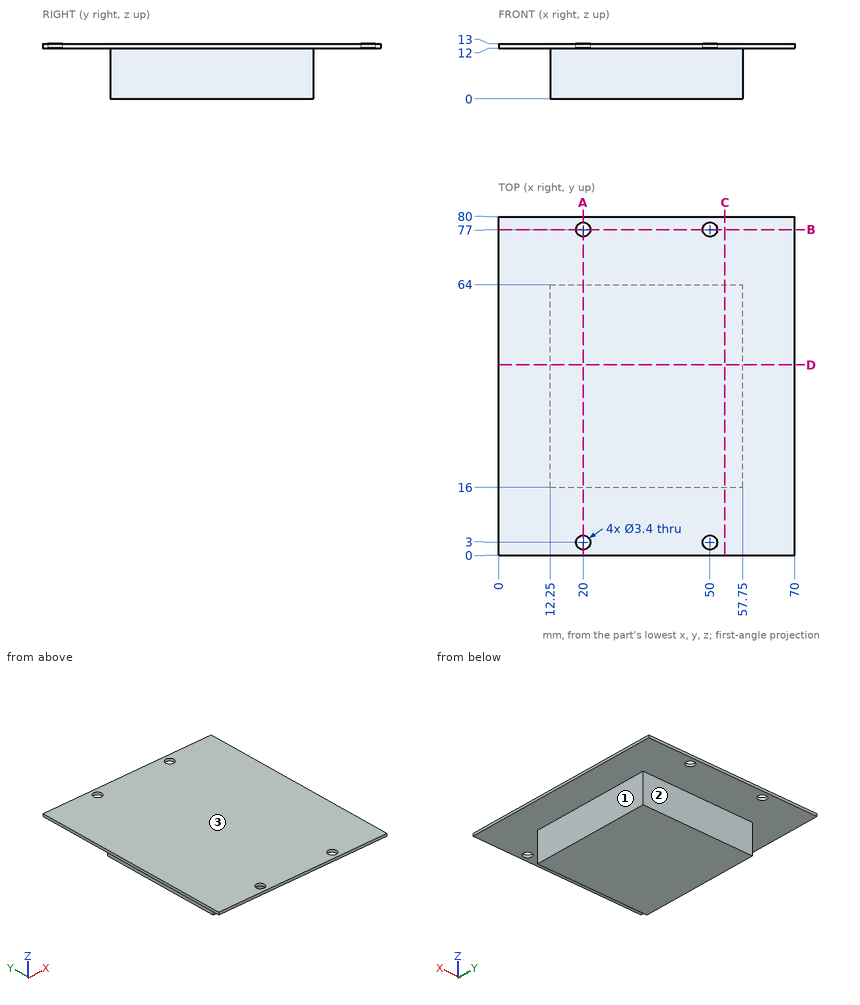
Study the drawing (mm; zero at the part's minimum x, y, z) and answer. A direction names the side the tool comes from. Round coordinates to 2 decimals unless told otherwise and drop trailing zeros. Order: outer loops, then holes, each group sorted by start corner. A loop starts at its lowest first (then second) coordinate and runs counter-clockwise, first axis right, second up. Notation, with made-up numbers: (80, -39) - (129, -39) arc R29 cw to (129, -1) - close; hole circle Ø6 at (70.25, -18.75). An arc over 180 degrees is marked (long way). Use one line per item in the form item = value. Start each with the question number.
(1) The part is cut by section B-B (y = 77). Give the vertices of the cut face in (x, z).
(2) The part is cut by section D-D (y = 45). Give the vertices of the cut face in (x, z).
(3) Flat-ended cylindrical pins translate along their axes: pin 1 Ø3.5 at (y, z) = (35, 4.5) entering from +X; pin 2 Ø6 at (y, z) = (43.5, 5.5) entering from -X; pin 3 Ø6 at (x, z) = (24.5, 8.5) entering from -Y; pin 4 Ø3 at (x, y) = (20, 77) entering from -Z. Find the tip coordinate at first contact, or state that the pin passes through.
(4) The part is cut by section C-C (x = 53.5). Give the vertices of the cut face in (y, z).
(5) The part is cut by section A-A (x = 20). Give the vertices of the cut face in (y, z), then the cut area to 3 significant figures.
(6) For the marked faces 1, 2 and 3, determine the directions among +Z, -Z, +X, -X, +Y, -Y from which every point of the face is accessible in a straight line to the end or side of a thin tool.
(7) Find the intervals of material crossed by line 1 along Y through (x, z) = (50, 12.3); line 2 along X through (y, z) = (77, 12.5); line 3 along X through (y, z) = (18, 2.25), in increasing order. Write a range as from..to.
Checked values:
q1.outline = (0, 12) - (18.3, 12) - (18.3, 13) - (0, 13) - close; (21.7, 12) - (48.3, 12) - (48.3, 13) - (21.7, 13) - close; (51.7, 12) - (70, 12) - (70, 13) - (51.7, 13) - close
q2.outline = (0, 12) - (12.25, 12) - (12.25, 0) - (57.75, 0) - (57.75, 12) - (70, 12) - (70, 13) - (0, 13) - close
q3.pin_1 = 57.75
q3.pin_2 = 12.25
q3.pin_3 = 16
q3.pin_4 = through
q4.outline = (0, 12) - (16, 12) - (16, 0) - (64, 0) - (64, 12) - (80, 12) - (80, 13) - (0, 13) - close
q5.outline = (0, 12) - (1.3, 12) - (1.3, 13) - (0, 13) - close; (4.7, 12) - (16, 12) - (16, 0) - (64, 0) - (64, 12) - (75.3, 12) - (75.3, 13) - (4.7, 13) - close; (78.7, 12) - (80, 12) - (80, 13) - (78.7, 13) - close
q5.area = 649 mm^2
q6.face_1 = -Z, +X, +Y, -Y
q6.face_2 = -Z, +X, -X, +Y
q6.face_3 = +Z, +X, -X, +Y, -Y
q7.line_1 = 0..1.3, 4.7..75.3, 78.7..80
q7.line_2 = 0..18.3, 21.7..48.3, 51.7..70
q7.line_3 = 12.25..57.75
